Verification items for the finished model (mm, model axes). A direction names the side the tool comes from. Coordinates: 2 decimals unless noted, no trailing zeros. Loops run counter-clockwise (first coordinate to the right, second up) from the corner with the lowest first, then second, coordinate; pieces in that order, holes last. Notation, with made-up numbers: (24.5, 76.5) -> (47.5, 76.5) arc R24 ccw to (47.5, 112.5) -> close; hole circle Ø11 at (89.25, 64.5). An arc over 180 degrees is marked (long way). Answer as a JSON object with one key per item and string values. Group by question number.
Q1. Cross-section at A-A on z = 4.5. Record the boundary of the cut face in (x, y), and give its area (3 significant figures).
Q2. Cross-section at C-C on x = 3. Record the boundary of the cut face in (y, z).
Q3. Gauge pin test, flat ends, axial feed: pin 1 Ø12 at (y, z) = (-4, -9) entering from -X; pin 2 Ø4 at (y, z) = (-7.5, 10.5) entering from +X; pin 3 Ø3 at (y, z) = (-14, 7.5) entering from +X. Record the tip position at first contact, or that the pin passes through.
Q4. Scan lines: L1, parallel to X at y = -6, z = 9.5; L2, parallel to X at y = -4, z = 9; L3, parallel to X at y = -1.25, z = -10.5. Record each from-to range of solid material in increasing order.
Q5. Cross-section at B-B on z = -12. Record the boundary of the cut face in (x, y), and give its area (3 significant figures).
Q6. Release check for a two-part mould opening along X. For faces 1 (the flat face through (0, 0, -1)), 2 (the flat face through (-6, -10, 0)), 3 (the cylindrical face through (-6.6, -10.14, 7.19)) record: released by +X, released by -X, zero draft, split by the parting line, or undercut.
Q7. Set-up check for faces 4 (the cylindrical face through (6.43, -10.14, 6.98)), 5 (the flat face through (0, -20, -1)): record each of +Z, -Z, +X, -X, +Y, -Y from which the full face is reachable in a straight line by a thin tool's end or side.
```python
from build123d import *

# Parameters (mm, degrees)
F0_W     = 24
F0_H     = 30
F1_DEPTH = 20
F3_DEPTH = 25
F5_DEPTH = 25


with BuildPart() as f1:
    # F0 (on Front) → F1 (new body)
    with BuildSketch(Plane.XZ):
        Rectangle(F0_W, F0_H)
    extrude(amount=F1_DEPTH)

    # F2 (on face) → F3 (cut)
    with BuildSketch(Plane.XZ.offset(20)):
        with BuildLine():
            ThreePointArc((-12, 15), (-6.516982, 7.086415), (0, 0))
            ThreePointArc((0, 0), (6.516982, 7.086415), (12, 15))
            Line((12, 15), (-12, 15))
        make_face()
    extrude(amount=-F3_DEPTH, mode=Mode.SUBTRACT)

    # F4 (on face) → F5 (cut)
    with BuildSketch(Plane.XZ.offset(20)):
        Polygon((12, 15), (0, -15), (12, -15), align=None)
        Polygon((0, -15), (-12, 15), (-12, -15), align=None)
    extrude(amount=-F5_DEPTH, mode=Mode.SUBTRACT)


solid = f1.part
```
Computed values:
{
 "1": {"outline": "(-7.8, -20) -> (-4.34, -20) -> (-4.34, 0) -> (-7.8, 0) -> close; (4.34, -20) -> (7.8, -20) -> (7.8, 0) -> (4.34, 0) -> close", "area": "138 mm²"},
 "2": {"outline": "(-20, -7.5) -> (0, -7.5) -> (0, 3.02) -> (-20, 3.02) -> close"},
 "3": {"pin 1": "stops at x = -4.8", "pin 2": "stops at x = 11", "pin 3": "stops at x = 9.6"},
 "4": {"L1": "x = -9.8 to -8.36, 8.36 to 9.8", "L2": "x = -9.6 to -7.99, 7.99 to 9.6", "L3": "x = -1.8 to 1.8"},
 "5": {"outline": "(-1.2, -20) -> (1.2, -20) -> (1.2, 0) -> (-1.2, 0) -> close", "area": "48.0 mm²"},
 "6": {"face 1": "zero draft", "face 2": "released by -X", "face 3": "undercut"},
 "7": {"face 4": "+Z, +Y, -Y", "face 5": "+Z, -Z, +X, -X, -Y"}
}
